```python
from build123d import *

# Parameters (mm, degrees)
PAD002_DEPTH = 8
SKETCH001_R  = 1.4
PAD001_DEPTH = 5
SKETCH_R     = 1.5
PAD_DEPTH    = 8


with BuildPart() as pad002:
    # Sketch002 → Pad002 (new body)
    with BuildSketch(Plane(origin=(-6, 10, 4), x_dir=(1, 0, 0), z_dir=(0, -1, 0))):
        Polygon((2, 4.1), (3, 3.52265), (4, 4.1), (5, 3.52265), (6, 4.1), (7, 3.52265), (8, 4.1), (9, 3.52265), (10, 4.1), (10, 5.1), (2, 5.1), align=None)
    extrude(amount=PAD002_DEPTH)


with BuildPart() as fusion:
    # Sketch001 → Pad001 (new body, symmetric)
    with BuildSketch(Plane.YZ):
        with Locations((6, 4)):
            Circle(SKETCH001_R)
    extrude(amount=PAD001_DEPTH, both=True)

    # Fusion: union Pad002
    add(pad002.part)


with BuildPart() as cut:
    # Sketch → Pad (new body)
    with BuildSketch(Plane.XY):
        with BuildLine():
            ThreePointArc((5, 12), (0, 17), (-5, 12))
            Line((-5, 12), (-5, 0))
            ThreePointArc((-5, 0), (0, -5), (5, 0))
            Line((5, 12), (5, 0))
        make_face()
        with Locations((0, 12)):
            Circle(SKETCH_R, mode=Mode.SUBTRACT)
        Circle(SKETCH_R, mode=Mode.SUBTRACT)
    extrude(amount=PAD_DEPTH)

    # Cut: cut Fusion
    add(fusion.part, mode=Mode.SUBTRACT)


solid = cut.part
```
Geometry: final body of the model. Coordinates: model frame, mm. A direction names the side the tool comes from. Give positions to 0.01 mm unless a question says otherwise; leave off trailing zeros. Loops run counter-clockwise (first coordinate to the right, second up) from the corner with the lowest first, then second, coordinate; pieces in that order, holes last. Notation, with made-up numbers: (83.5, 7.5) - (107.5, 7.5) arc R32 ccw to (107.5, 36.5) - close; hole circle Ø4 at (20.5, 73.5). An arc over 180 degrees is marked (long way). Answer as CSV lines item,"result". Start each with the question number.
(1) Ray query, line 1 along Y through (x, z) = (0, 2.5); line 2 along Y through (x, z) = (-0.75, 6.25); line 3 along Z through (x, y) = (-2, 6.5). Return the intervals inside material, ascending. Write a range as [from, to].
(2) Section query A-A (z = 4). Output: boundary loops of the cut face in (x, y).
(3) Section query B-B (y = 6). Output: boundary loops of the cut face in (x, z), and give its area (3 significant figures).
(4) Reachability of faces 5 (the face through (0.07, 7.29, 3.46)), 6 (the face through (-2.59, 6.06, 7.76)) from +Z, -Z, +X, -X, +Y, -Y: full face, straight path, thin tool, end or side. Return the list, or none.
(5) Mould query, pull axis Y, two halves, no side actions, for faces 1 (the face through (5, 7.4, 4.8)), 2 (the face through (-0.59, 6.06, 7.76)), 3 (the face through (0, -5, 4)), 4 (the face through (0, 17, 4)). Classes: +Y half, -Y half, draft (parallel to the pull), parting line (faces both ways), or undercut.
(6) Section query C-C (x = 2.5). Output: boundary loops of the cut face in (y, z), and give its area (3 significant figures).
(7) Section query D-D (z = 1.5). Output: boundary loops of the cut face in (x, y), and give its area (3 significant figures).
(8) Pin query (flat end, axial travel): P1, Ø6, axis at x = -1.5, y = 8.5, coming from the -Z side; P2, Ø1.5, axis at x = 2, z = 5, coming from the -Y side; P3, Ø2.5, axis at y = 6, z = 4, coming from the +X side; P4, Ø3, axis at x = 3.5, z = 1.5, coming from the -Y side. Return the tip coordinate at first contact, or that it passes through.
Worked answers:
1,line 1,"y = [-5, -1.5], [1.5, 10.5], [13.5, 17]"
1,line 2,"y = [-4.94, -1.3], [1.3, 10.7], [13.3, 16.94]"
1,line 3,"z = [0, 2.69], [5.31, 8]"
2,outline,"(-5, 0) arc R5 ccw to (5, 0) - (5, 4.6) - (-5, 4.6) - close; (-5, 7.4) - (5, 7.4) - (5, 12) arc R5 ccw to (-5, 12) - close; hole circle Ø3 at (0, 0); hole circle Ø3 at (0, 12)"
3,outline,"(-5, 0) - (5, 0) - (5, 2.6) - (-5, 2.6) - close; (-5, 5.4) - (5, 5.4) - (5, 8) - (3.83, 8) - (3, 7.52) - (2.17, 8) - (1.83, 8) - (1, 7.52) - (0.17, 8) - (-0.17, 8) - (-1, 7.52) - (-1.83, 8) - (-2.17, 8) - (-3, 7.52) - (-3.83, 8) - (-5, 8) - close"
3,area,"50.4 mm^2"
4,face 5,"+X, -X"
4,face 6,"+Z"
5,face 1,"draft"
5,face 2,"undercut"
5,face 3,"-Y half"
5,face 4,"+Y half"
6,outline,"(-4.33, 0) - (16.33, 0) - (16.33, 8) - (10, 8) - (10, 7.81) - (2, 7.81) - (2, 8) - (-4.33, 8) - close; hole circle Ø2.8 at (6, 4)"
6,area,"158 mm^2"
7,outline,"(-5, 0) arc R5 ccw to (5, 0) - (5, 12) arc R5 ccw to (-5, 12) - close; hole circle Ø3 at (0, 0); hole circle Ø3 at (0, 12)"
7,area,"184 mm^2"
8,P1,"stops at z = 0"
8,P2,"stops at y = -4.84"
8,P3,"passes through"
8,P4,"stops at y = -4.58"
